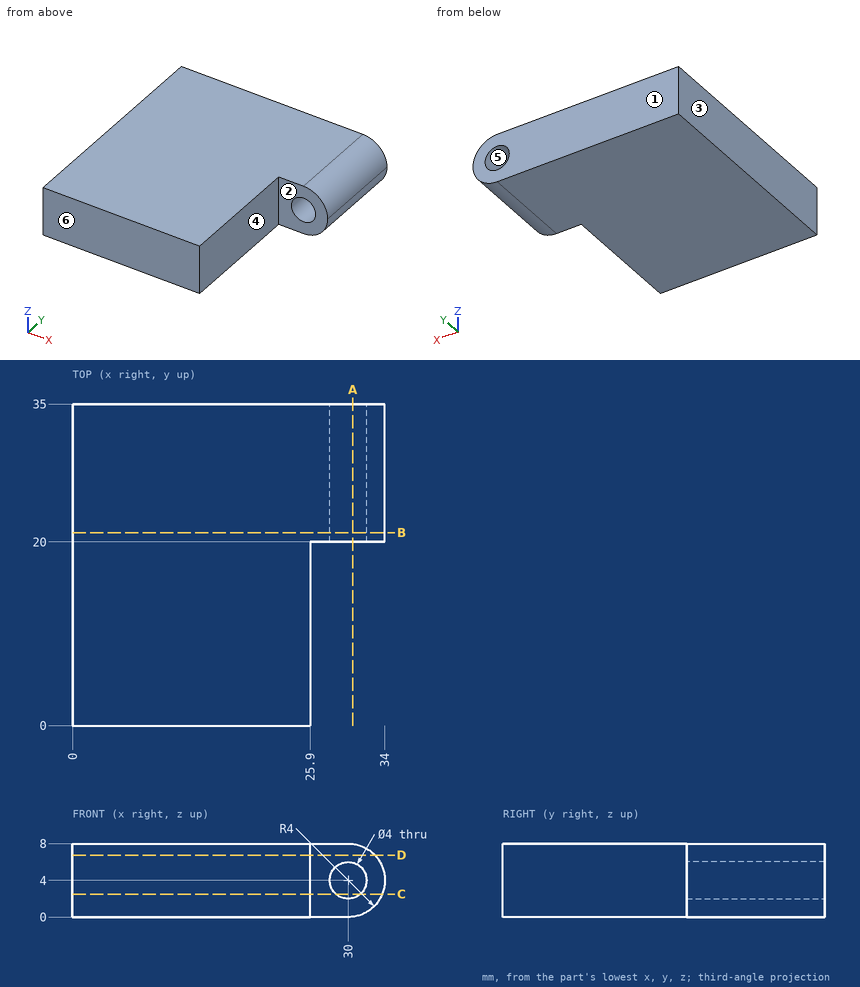
Here's the drawing with two shaded views (mm, measured from the low corner). I have some questions. A direction names the side the tool comes from. Round coordinates to 2 decimals unless told otherwise and drop trailing zeros. Order: outer loops, then holes, each group sorted by start corner. A loop starts at its lowest first (then second) coordinate and runs counter-clockwise, first axis right, second up. Notation, with made-up numbers: (53, 58) -> (97, 58) arc R27 cw to (97, 77) -> close; hole circle Ø10 at (-17.75, 23). An arc over 180 degrees is marked (long way). Use a Markdown table: item, result. Add a question column.
(1) Suppose I cut it at C-C, the plane z = 2.5. Please give me the cut outline in (x, y), and give its area (3 significant figures).
(2) If we mould it in two halves opening along X, with no side actions, what happens to the marked faces 3, 4, 5 and 6? For each: released by +X, released by -X, zero draft, split by the parting line, or undercut.
(3) For pin 1 Ø3 at (x, z) = (30, 4) entering from +Y; pin 2 Ø3 at (y, z) = (24, 7) entering from +X; pin 3 Ø10 at (x, y) = (22.5, 15) entering from -Z; pin 4 Ø2 at (y, z) = (28, 2) entering from +X, each with a flat end and sliding along its axis, tell me the tip position at first contact or that it passes through.
(4) Suppose I cut it at A-A, the plane x = 30.5. Please give me the cut outline in (y, z), and give its area (3 significant figures).
(5) For the marked faces 1 and 2, which set-ups out of +Z, -Z, +X, -X, +Y, -Y let a thin tool reach every point of the face, with its end or its side?
(6) I need wall thicknesses on line 1 along X through (y, z) = (28.5, 4); line 2 along X through (y, z) = (6, 7.5); line 3 along Y through (x, z) = (29, 6.25). Which ranges of each line are inside material? Lowest first, please.
(7) Suppose I cut it at B-B, the plane y = 21. Please give me the cut outline in (x, z).
(8) Suppose I cut it at D-D, the plane z = 6.75. Please give me the cut outline in (x, y), and give its area (3 significant figures).
Verdict:
| question | item | result |
|---|---|---|
| 1 | outline | (0, 0) -> (25.9, 0) -> (25.9, 20) -> (28.68, 20) -> (28.68, 35) -> (0, 35) -> close; (31.32, 20) -> (33.71, 20) -> (33.71, 35) -> (31.32, 35) -> close |
| 1 | area | 984 mm2 |
| 2 | face 3 | released by -X |
| 2 | face 4 | released by +X |
| 2 | face 5 | undercut |
| 2 | face 6 | zero draft |
| 3 | pin 1 | through |
| 3 | pin 2 | x = 33.71 |
| 3 | pin 3 | z = 0 |
| 3 | pin 4 | x = 33.87 |
| 4 | outline | (20, 0.03) -> (35, 0.03) -> (35, 2.06) -> (20, 2.06) -> close; (20, 5.94) -> (35, 5.94) -> (35, 7.97) -> (20, 7.97) -> close |
| 4 | area | 61.0 mm2 |
| 5 | face 1 | +Z, -Z, +X, -X, +Y |
| 5 | face 2 | +Z, -Z, +X, -Y |
| 6 | line 1 | 0 to 28, 32 to 34 |
| 6 | line 2 | 0 to 25.9 |
| 6 | line 3 | 20 to 35 |
| 7 | outline | (0, 0) -> (30, 0) arc R4 ccw to (30, 8) -> (0, 8) -> close; hole circle Ø4 at (30, 4) |
| 8 | outline | (0, 0) -> (25.9, 0) -> (25.9, 20) -> (32.9, 20) -> (32.9, 35) -> (0, 35) -> close |
| 8 | area | 1,010 mm2 |
